Model file for the job. Use its own axes, mm. A direction names the side the tool comes from. Round coordinates to 2 decimals unless told otherwise and drop trailing zeros. Order: outer loops, then holes, each group sorted by start corner. A loop starts at its lowest first (then second) coordinate and runs counter-clockwise, first axis right, second up. Notation, with made-up numbers: (80, -29.5) -> (100, -29.5) arc R34 cw to (100, 5.5) -> close; hole circle Ø7 at (51.25, 45). An arc over 180 degrees is marked (long way). Use CSV: the item, a comma, the result in double quotes.
```python
from build123d import *

# Parameters (mm, degrees)
F1_DEPTH = 25


# Not quite as in the source:
# - ends of sketch curves that miss each other by under 0.0002 mm in the source are joined


with BuildPart() as f1:
    # F0 (on Top) → F1 (new body)
    with BuildSketch(Plane.XY):
        with BuildLine():
            ThreePointArc((48.1663785379, 9.9999997765), (33.5940436684, 12.9051702933), (21.2498728844, 21.1764704896))
            ThreePointArc((21.2498728844, 21.1764704896), (-30, 6.96e-08), (21.2498727861, -21.1764705882))
            ThreePointArc((21.2498727861, -21.1764705882), (33.5940435271, -12.9051704831), (48.1663783152, -10))
            Line((48.1663783152, -10), (75, -10))
            ThreePointArc((75, -10), (84.9999997765, 0), (75, 9.9999997765))
            Line((75, 9.9999997765), (48.1663785379, 9.9999997765))
        make_face()
        with BuildLine():
            ThreePointArc((14.1421356237, -5), (-15, 0), (14.1421356237, 5))
            Line((14.1421356237, 5), (75, 5))
            ThreePointArc((75, 5), (80, 0), (75, -5))
            Line((75, -5), (14.1421356237, -5))
        make_face(mode=Mode.SUBTRACT)
    extrude(amount=F1_DEPTH)


solid = f1.part
```
Q1. Cut at B-B (y = 0). Give the cut face in (x, z).
From the geometry:
outline,"(-30, 0) -> (-15, 0) -> (-15, 25) -> (-30, 25) -> close; (80, 0) -> (85, 0) -> (85, 25) -> (80, 25) -> close"
Q2. Which spindle directions (+Z, -Z, +X, -X, +Y, -Y) get a long thin tool onto all of the face, cutting with end or side? Do faces 1 (the flat face through (14, -6, 25)), 2 (the cylindrical face through (85, 0, 12)), 3 (the flat face through (61, -10, 12)), 4 (the flat face through (62, 10, 12)), 5 (the flat face through (44, 5, 12)). Say none if no direction does.
From the geometry:
face 1,"+Z, +X, -X, +Y, -Y"
face 2,"+Z, -Z, +X"
face 3,"+Z, -Z, +X, -Y"
face 4,"+Z, -Z, +X, +Y"
face 5,"+Z, -Z"
Q3. Probe line 1 along Y through (x, z) = (0, 6.25); line 2 along Y through (x, z) = (54, 1.5); line 3 along X through (y, z) = (5.5, 3). List the from-to ranges inside material, lowest first.
From the geometry:
line 1,"y = -30 to -15, 15 to 30"
line 2,"y = -10 to -5, 5 to 10"
line 3,"x = -29.49 to -13.96, 13.96 to 83.35"
Q4. Pin check, flat tips, straight feed: pin 1 (1 mm diameter, centred on y = -19.5, z = 5, fed in from -X); pin 2 (12.5 mm diameter, centred on x = 47.5, z = 8.5, fed in from -Y); pin 3 (3 mm diameter, centred on x = 61, z = 13, fed in from -Y). Stop position of each tip, or through.
From the geometry:
pin 1,"stops at x = -23.22"
pin 2,"stops at y = -10.63"
pin 3,"stops at y = -10"
Q5. Cut at D-D (y = -19). Give the cut face in (x, z), plus the area to 3 significant figures.
From the geometry:
outline,"(-23.22, 0) -> (23.61, 0) -> (23.61, 25) -> (-23.22, 25) -> close"
area,"1,170 mm²"
Q6. Cut at A-A (x = 0). Give the cut face in (y, z).
From the geometry:
outline,"(-30, 0) -> (-15, 0) -> (-15, 25) -> (-30, 25) -> close; (15, 0) -> (30, 0) -> (30, 25) -> (15, 25) -> close"
Q7. Cut at C-C (z = 5.5). Give the cut face in (x, y).
From the geometry:
outline,"(21.25, -21.18) arc R38 cw to (48.17, -10) -> (75, -10) arc R10 ccw to (75, 10) -> (48.17, 10) arc R38 cw to (21.25, 21.18) arc R30 ccw (long way) to start; hole (14.14, -5) -> (75, -5) arc R5 ccw to (75, 5) -> (14.14, 5) arc R15 ccw (long way) to start"
Q8. Mould opens along X. For faces 6 (the flat face through (14, -6, 0)), 7 (the cylindrical face through (33.788, 12.825, 12.325)), 8 (the cylindrical face through (80, 0, 12)) say: +X half, -X half, draft (parallel to the pull), parting line (faces both ways), or undercut.
From the geometry:
face 6,"draft"
face 7,"+X half"
face 8,"undercut"
